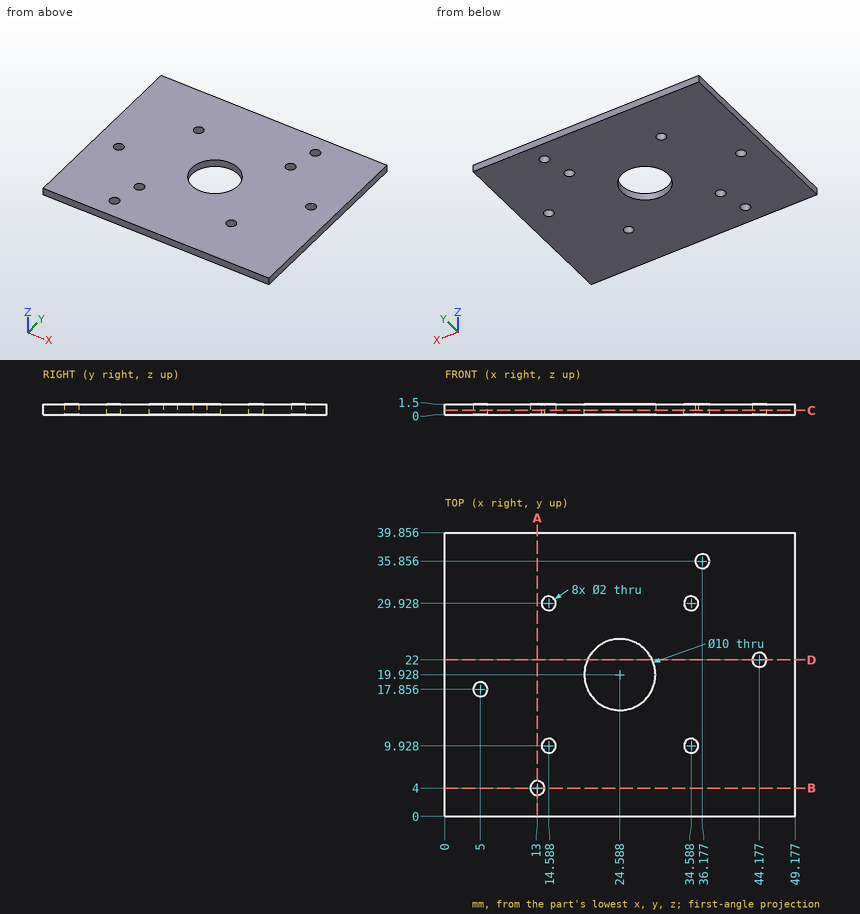
Answer from the drawing. Dimensions are ordinates in mm from the lowest x, y and z of the part. Give positions to 0.01 mm unless a question says otherwise; leave off trailing zeros. Order: outer loops, then holes, each group sorted by start corner. A loop starts at its lowest first (then second) coordinate and runs counter-clockwise, first axis right, second up. Notation, with made-up numbers: (-13.5, -30) -> (-4.5, -30) arc R14 cw to (-4.5, -22) -> close; hole circle Ø1 at (-13, 12.25). An arc over 180 degrees is marked (long way). One line per item, written item: value.
Item 1: Straight lines are drawn through the part: probe 1 along X at (y, z) = (30, 0.2) (1 decimal); probe 2 along Y at (x, z) = (34, 1.3) (1 decimal); probe 3 along X at (y, z) = (18.5, 0.4) (1 decimal). For each, find the intervals that lie inside material, in ascending order.
Answer sheet:
probe 1: 0 to 13.6, 15.6 to 33.6, 35.6 to 49.2
probe 2: 0 to 9.1, 10.7 to 29.1, 30.7 to 39.9
probe 3: 0 to 4.2, 5.8 to 19.8, 29.4 to 49.2
Item 2: Find section A-A, the plane x = 13. Give the vertices of the cut face in (y, z).
Answer sheet:
outline: (0, 0) -> (3, 0) -> (3, 1.5) -> (0, 1.5) -> close; (5, 0) -> (39.86, 0) -> (39.86, 1.5) -> (5, 1.5) -> close
Item 3: Find section C-C, the plane z = 0.6. State how many separate pieces and enclosed holes the cut face has, plus the area to 3 significant figures.
Answer sheet:
separate pieces: 1
enclosed holes: 9
area: 1,860 mm²
Item 4: Find section B-B, the plane y = 4. Give the vertices of the cut face in (x, z).
Answer sheet:
outline: (0, 0) -> (12, 0) -> (12, 1.5) -> (0, 1.5) -> close; (14, 0) -> (49.18, 0) -> (49.18, 1.5) -> (14, 1.5) -> close
Item 5: Find section D-D, the plane y = 22. Give the vertices of the cut face in (x, z).
Answer sheet:
outline: (0, 0) -> (20.04, 0) -> (20.04, 1.5) -> (0, 1.5) -> close; (29.14, 0) -> (43.18, 0) -> (43.18, 1.5) -> (29.14, 1.5) -> close; (45.18, 0) -> (49.18, 0) -> (49.18, 1.5) -> (45.18, 1.5) -> close
